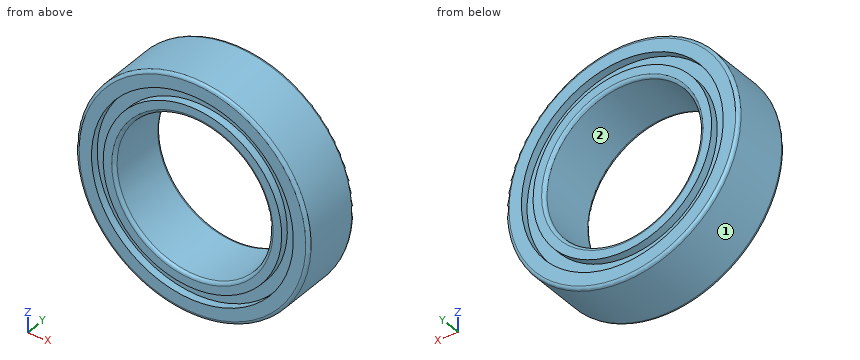
from build123d import *

# Parameters (mm, degrees)
BOSS_EXTRUDE1_DEPTH      = 2
BOSS_EXTRUDE1_DEPTH_BACK = 2
SKETCH1_R                = 7.5
SKETCH1_R_2              = 5
SKETCH2_R                = 6.5
SKETCH2_R_2              = 5.75
CUT_EXTRUDE1_DEPTH       = 0.5
FILLET1_R                = 0.2


with BuildPart() as part:
    # Sketch1 → Boss-Extrude1 (new, two sides: drawn at the far end of the back side and taken through both)
    with BuildSketch(Plane(origin=(0, 0, 0), x_dir=(1, 0, 0), z_dir=(0, 1, 0)).offset(-BOSS_EXTRUDE1_DEPTH_BACK)):
        with Locations(Location((0, 0, 0), (0, 0, 270))):
            Circle(SKETCH1_R)
        with Locations(Location((0, 0, 0), (0, 0, 270))):
            Circle(SKETCH1_R_2, mode=Mode.SUBTRACT)
    extrude(amount=BOSS_EXTRUDE1_DEPTH + BOSS_EXTRUDE1_DEPTH_BACK)

    # Sketch2 → Cut-Extrude1 (cut)
    with BuildSketch(Plane(origin=(0, 2, 0), x_dir=(1, 0, 0), z_dir=(0, 1, 0))):
        with Locations(Location((0, 0, 0), (0, 0, 270))):
            Circle(SKETCH2_R)
        with Locations(Location((0, 0, 0), (0, 0, 270))):
            Circle(SKETCH2_R_2, mode=Mode.SUBTRACT)
    cut_extrude1 = extrude(amount=-CUT_EXTRUDE1_DEPTH, mode=Mode.SUBTRACT)

    # Mirror2: Cut-Extrude1 across plane
    add(cut_extrude1.mirror(Plane.ZX), mode=Mode.SUBTRACT)

    # Fillet1
    fillet1_edges = [part.edges().sort_by_distance(p)[0] for p in [
        (0, -2, -7.5),
        (0, -2, -5),
        (0, 2, -7.5),
        (0, 2, -5),
    ]]
    fillet(fillet1_edges, radius=FILLET1_R)


solid = part.part
Build history of the part. All positions in model axes, mm. Face numbers are marked on the shaded views. Give positions to 0.01 mm unless a question says otherwise; leave off trailing zeros. Order: outer loops, then holes, each group sorted by start corner. A loop starts at its lowest first (then second) coordinate and runs counter-clockwise, first axis right, second up. Notation, with made-up numbers: M -23.75,56.5 L 0.25,56.5 A29 cw 0.25,89.5 Z; hole C 75,74 d10. An arc over 180 degrees is marked long. Put each result on its own line as item: value.
Item 1: Cut at C-C on y = 0.15. Write the cut outline in (x, z), then the cut area to 3 significant figures.
Results are:
outline: C 0,0 d15; hole C 0,0 d10
area: 98.2 mm2
Item 2: Wall check: probe 1 along X at (y, z) = (0.5, 0); probe 2 along Z at (x, y) = (-1.25, 1.7); probe 3 along X at (y, z) = (1.75, 0). Give the ranges that are in metal, low to high.
Results are:
probe 1: -7.5 to -5, 5 to 7.5
probe 2: -7.4 to -6.38, -5.61 to -4.84, 4.84 to 5.61, 6.38 to 7.4
probe 3: -7.5 to -6.5, -5.75 to -5, 5 to 5.75, 6.5 to 7.5
Item 3: Pull direction X, two halves, no side cores. Call the marked faces 1 and 2: +X half, -X half, draft (parallel to the pull), parting line (faces both ways), or undercut.
Results are:
face 1: parting line
face 2: undercut
